The model under review builds one solid part; all positions refer to its coordinate system, in mm. Face numbers are marked on the shaded views. A direction names the side the tool comes from. Coordinates: 2 decimals unless noted, no trailing zeros. Loops run counter-clockwise (first coordinate to the right, second up) from the corner with the lowest first, then second, coordinate; pieces in that order, holes last. Notation, with made-up numbers: M -6,-5 L 18,-5 A18 cw 18,11 Z; hole C 79.25,82 d7. An arc over 180 degrees is marked long. Use CSV: the item, a comma, the result in double quotes. Start each with the question number.
1. For L1, parallel to Z at x = 0, y = -60; L2, parallel to Z at x = 0, y = 12; L3, parallel to Z at x = 0, y = -5, list the stretches that pass through material, from the lowest coordinate up.
2. Tool access review of the marked faces 1 and 2: name each direction out of +Z, -Z, +X, -X, +Y, -Y from which nothing blocks a thin tool from reaching the whole face with its end or side.
3. Clearance check with flat-ended pins moving along their axes: P1, Ø1, axis at y = -15.5, z = 64, coming from the -X side; P2, Ø6, axis at x = -46.5, z = -20.5, coming from the +Y side; P3, Ø10, axis at x = -17, y = -45.5, coming from the -Z side; P4, Ø20.5, axis at x = 0, z = 0, coming from the -Y side. State where each tip first meets the part, or that it passes through.
4. Draft analysis for pull direction Z (two halves, no side actions). For the marked faces 3, 4, 5 and 6, state which applies: +Z half, -Z half, draft (parallel to the pull), parting line (faces both ways), or undercut.
5. Add section C-C, the plane y = 13.5. Write out the cut boundary in (x, z).
from build123d import *

# Parameters (mm, degrees)
F0_R          = 86.6272823849
F1_DEPTH      = 25.4
F2_R          = 86.6272823849
F2_R_2        = 67.8769245924
F3_DEPTH      = 76.2
F4_R          = 34.1816109176
F4_R_2        = 17.2424518984
F5_DEPTH      = 50.8
F5_DEPTH_BACK = 50.8
F6_R          = 16.8190059926
F7_DEPTH      = 50.8
F8_R          = 12.7
F9_R          = 12.7


with BuildPart() as f1:
    # F0 (on Front) → F1 (new body)
    with BuildSketch(Plane.XZ):
        Circle(F0_R)
    extrude(amount=F1_DEPTH)

    # F2 (on face) → F3 (join)
    with BuildSketch(Plane.XZ.offset(25.4)):
        Circle(F2_R)
        Circle(F2_R_2, mode=Mode.SUBTRACT)
    extrude(amount=F3_DEPTH)

    # F4 (on face) → F5 (join, two sides)
    with BuildSketch(Plane.XZ.offset(25.4)) as f5_sk:
        Circle(F4_R)
        Circle(F4_R_2, mode=Mode.SUBTRACT)
    extrude(amount=F5_DEPTH)
    extrude(f5_sk.sketch, amount=-F5_DEPTH_BACK)

    # F6 (on face) → F7 (cut)
    with BuildSketch(Plane.XZ.offset(25.4)):
        Circle(F6_R)
    extrude(amount=-F7_DEPTH, mode=Mode.SUBTRACT)

    # F8
    f8_edges = [f1.edges().sort_by_distance(p)[0] for p in [
        (-67.876925, -101.6, 0),
    ]]
    fillet(f8_edges, radius=F8_R)

    # F9
    f9_edges = [f1.edges().sort_by_distance(p)[0] for p in [
        (-67.876925, -25.4, 0),
        (-34.181611, -25.4, 0),
    ]]
    fillet(f9_edges, radius=F9_R)


solid = f1.part
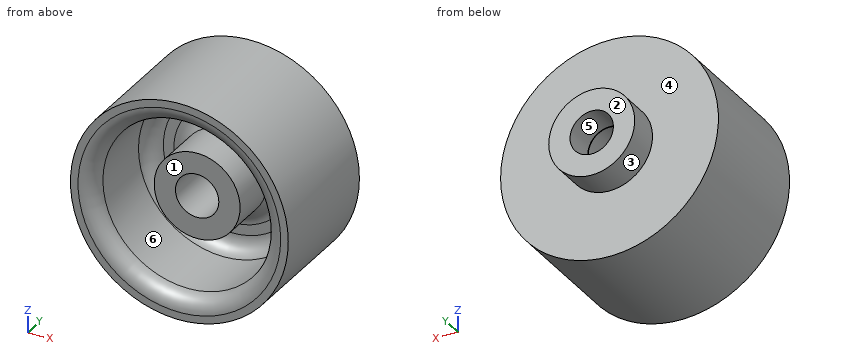
Computed:
1,L1,"z = -86.63 to -67.88, -34.18 to -17.24, 17.24 to 34.18, 67.88 to 86.63"
1,L2,"z = -34.18 to -17.24, 17.24 to 34.18"
1,L3,"z = -86.63 to -16.82, 16.82 to 86.63"
2,face 1,"-Y"
2,face 2,"+Z, -Z, +X, -X, +Y"
3,P1,"stops at x = -58.92"
3,P2,"stops at y = 0"
3,P3,"stops at z = -85.79"
3,P4,"passes through"
4,face 3,"parting line"
4,face 4,"draft"
4,face 5,"undercut"
4,face 6,"undercut"
5,outline,"C 0,0 d68.36; hole C 0,0 d34.48"
